from build123d import *

# Parameters (mm, degrees)
F1_W           = 497
F1_H           = 754
F2_DEPTH       = 18
F5_D           = 8
F5_DEPTH       = 28
F5_TIP         = 2.4034424761
F5_ON_F4_D     = 8
F5_ON_F4_DEPTH = 28
F5_ON_F4_TIP   = 2.4034424761
F7_D           = 5
F7_DEPTH       = 34
F7_TIP         = 1.5021515476
F9_D           = 15
F9_DEPTH       = 15
F9_TIP         = 4.5064546427


with BuildPart() as f2:
    # F1 (on offset) → F2 (new body)
    with BuildSketch(Plane.XZ.offset(283)):
        with Locations((1.2963563204, 75.9517796117)):
            Rectangle(F1_W, F1_H)
    extrude(amount=F2_DEPTH)

    # F5
    with Locations(Plane.XY.offset(452.9517796117)):
        with Locations((-187.2036436796, -292), (-127.2036436796, -292), (129.7963563204, -292), (189.7963563204, -292)):
            Hole(F5_D / 2, depth=F5_DEPTH)
            with Locations((0, 0, -(F5_DEPTH + F5_TIP / 2))):  # 118° drill point
                Cone(0, F5_D / 2, F5_TIP, mode=Mode.SUBTRACT)

    # F5 on F4
    with Locations(Plane(origin=(0, 0, -301.0482203883), x_dir=(1, 0, 0), z_dir=(0, 0, -1))):
        with Locations((-187.2036436796, 292), (-127.2036436796, 292), (129.7963563204, 292), (189.7963563204, 292)):
            Hole(F5_ON_F4_D / 2, depth=F5_ON_F4_DEPTH)
            with Locations((0, 0, -(F5_ON_F4_DEPTH + F5_ON_F4_TIP / 2))):  # 118° drill point
                Cone(0, F5_ON_F4_D / 2, F5_ON_F4_TIP, mode=Mode.SUBTRACT)

    # F7
    with Locations(Plane(origin=(-247.2036436796, 0, 0), x_dir=(0, -1, 0), z_dir=(-1, 0, 0))):
        with Locations((292, 372.9517796117), (292, 75.9517796117), (292, -221.0482203883)):
            Hole(F7_D / 2, depth=F7_DEPTH)
            with Locations((0, 0, -(F7_DEPTH + F7_TIP / 2))):  # 118° drill point
                Cone(0, F7_D / 2, F7_TIP, mode=Mode.SUBTRACT)

    # F9
    with Locations(Plane(origin=(0, -283, 0), x_dir=(-1, 0, 0), z_dir=(0, 1, 0))):
        with Locations((-189.7963563204, 418.9517796117), (187.2036436796, 418.9517796117), (187.2036436796, -267.0482203883), (-189.7963563204, -267.0482203883)):
            Hole(F9_D / 2, depth=F9_DEPTH)
            with Locations((0, 0, -(F9_DEPTH + F9_TIP / 2))):  # 118° drill point
                Cone(0, F9_D / 2, F9_TIP, mode=Mode.SUBTRACT)


solid = f2.part
Verification items for the finished model (mm, model axes). A direction names the side the tool comes from. Round coordinates to 2 decimals unless told otherwise and drop trailing zeros. Use one line per item in the form item = value.
1. Gauge pin test, flat ends, axial feed: pin 1 Ø3 at (y, z) = (-292, 75.95) entering from -X; pin 2 Ø6.5 at (x, y) = (129.8, -292) entering from +Z; pin 3 Ø2 at (x, y) = (-188.5, -293.5) entering from -Z. Record the tip position at first contact, or that the pin passes through.
A:
pin_1 = -212.6
pin_2 = 424.5
pin_3 = -259.91
2. Access from +Z, -Z, +X, -X, +Y, -Y to the whole of each face (thin tool, end or side, straight path). Record for faces 1 (the flat face through (-2, -292, 452.952)), 2 (the cylindrical face through (-188.83, -290.6, 411.63)).
A:
face_1 = +Z, +X, -X, +Y, -Y
face_2 = +Y
3. Scan lines: probe 1 along Z at (x, y) = (-231.5, -292); probe 2 along X at (y, z) = (-292, 431). Record each from-to range of solid material in increasing order.
A:
probe_1 = -301.05 to -223.55, -218.55 to 73.45, 78.45 to 370.45, 375.45 to 452.95
probe_2 = -247.2 to -191.2, -183.2 to -131.2, -123.2 to 125.8, 133.8 to 185.8, 193.8 to 249.8
4. Draft check along X on faces 3 (the flat face through (249.796, -292, 71)), 4 (the flat face through (-2, -301, 81)), 5 (the flat face through (-247.204, -292, 71)), 6 (the conical face through (190.16, -300.81, 421.75)). Enter one of: pulls with the +X half, pulls with the -X half, needs draft (parallel to the pull), parting line crosses it, or undercut.
A:
face_3 = pulls with the +X half
face_4 = needs draft
face_5 = pulls with the -X half
face_6 = undercut
